from build123d import *

# Parameters (mm, degrees)
SKETCH_1_R          = 1.5
EXTRUDE_1_DEPTH     = 2
EXTRUDE_2_DEPTH     = 17.8
EXTRUDE_3_DEPTH     = 1
CUT_EXTRUDE_START   = 1
CUT_EXTRUDE_1_DEPTH = 13
SKETCH_5_W          = 0.8
SKETCH_5_H          = 3.8
EXTRUDE_4_DEPTH     = 13
SKETCH_6_W          = 4
SKETCH_6_H          = 1
EXTRUDE_5_DEPTH     = 18


with BuildPart() as part:
    # 草图1 → 凸台-拉伸1 (new body)
    with BuildSketch(Plane(origin=(0, 0, 0), x_dir=(1, 0, 0), z_dir=(0, 1, 0))):
        with BuildLine():
            Line((-24.216959088, 1.570750156), (-14.242466434, 28.34905559))
            ThreePointArc((-14.242466434, 28.34905559), (-13.875866128, 28.821296411), (-13.305364415, 29))
            Line((-13.305364415, 29), (13.305364415, 29))
            ThreePointArc((13.305364415, 29), (13.875866128, 28.821296411), (14.242466434, 28.34905559))
            Line((14.242466434, 28.34905559), (24.216959088, 1.570750156))
            ThreePointArc((24.216959088, 1.570750156), (24.5, 0), (24.216959088, -1.570750156))
            Line((24.216959088, -1.570750156), (14.242466434, -28.34905559))
            ThreePointArc((14.242466434, -28.34905559), (13.875866128, -28.821296411), (13.305364415, -29))
            Line((13.305364415, -29), (-13.305364415, -29))
            ThreePointArc((-13.305364415, -29), (-13.875866128, -28.821296411), (-14.242466434, -28.34905559))
            Line((-14.242466434, -28.34905559), (-24.216959088, -1.570750156))
            ThreePointArc((-24.216959088, -1.570750156), (-24.5, 0), (-24.216959088, 1.570750156))
        make_face()
        with Locations((-20, 0)):
            Circle(SKETCH_1_R, mode=Mode.SUBTRACT)
        with Locations((20, 0)):
            Circle(SKETCH_1_R, mode=Mode.SUBTRACT)
    extrude(amount=EXTRUDE_1_DEPTH)

    # 草图2 → 凸台-拉伸2 (add)
    with BuildSketch(Plane.XZ):
        with BuildLine():
            Line((-13.3, -19.3), (-9.3, -23.3))
            Line((-9.3, -23.3), (9.3, -23.3))
            Line((9.3, -23.3), (13.3, -19.3))
            Line((13.3, -19.3), (13.3, 21.3))
            ThreePointArc((13.3, 21.3), (12.714213562, 22.714213562), (11.3, 23.3))
            Line((11.3, 23.3), (-11.3, 23.3))
            ThreePointArc((-11.3, 23.3), (-12.714213562, 22.714213562), (-13.3, 21.3))
            Line((-13.3, 21.3), (-13.3, -19.3))
        make_face()
    extrude(amount=EXTRUDE_2_DEPTH)

    # 草图4 → 凸台-拉伸3 (add)
    with BuildSketch(Plane(origin=(0, 2, 0), x_dir=(1, 0, 0), z_dir=(0, 1, 0))):
        with BuildLine():
            Line((-10.25, 27.15), (10.25, 27.15))
            ThreePointArc((10.25, 27.15), (13.078427125, 25.978427125), (14.25, 23.15))
            Line((14.25, 23.15), (14.25, -23.15))
            ThreePointArc((14.25, -23.15), (13.078427125, -25.978427125), (10.25, -27.15))
            Line((10.25, -27.15), (-10.25, -27.15))
            ThreePointArc((-10.25, -27.15), (-13.078427125, -25.978427125), (-14.25, -23.15))
            Line((-14.25, -23.15), (-14.25, 23.15))
            ThreePointArc((-14.25, 23.15), (-13.078427125, 25.978427125), (-10.25, 27.15))
        make_face()
    extrude(amount=EXTRUDE_3_DEPTH)

    # 草图3 → 切除-拉伸1 (cut)
    with BuildSketch(Plane(origin=(0, 2, 0), x_dir=(1, 0, 0), z_dir=(0, 1, 0)).offset(CUT_EXTRUDE_START)):
        with BuildLine():
            Line((-9, 20.034278181), (9, 20.034278181))
            Line((9, 20.034278181), (12, 17.034278181))
            Line((12, 17.034278181), (12, 4.034278181))
            ThreePointArc((12, 4.034278181), (11.707106781, 3.327171399), (11, 3.034278181))
            Line((11, 3.034278181), (-11, 3.034278181))
            ThreePointArc((-11, 3.034278181), (-11.707106781, 3.327171399), (-12, 4.034278181))
            Line((-12, 4.034278181), (-12, 17.034278181))
            Line((-12, 17.034278181), (-9, 20.034278181))
        make_face()
    extrude(amount=-CUT_EXTRUDE_1_DEPTH, mode=Mode.SUBTRACT)

    # 草图5 → 凸台-拉伸4 (add)
    with BuildSketch(Plane(origin=(0, -10, 0), x_dir=(1, 0, 0), z_dir=(0, 1, 0))):
        with Locations((-7, 9.698034266)):
            Rectangle(SKETCH_5_W, SKETCH_5_H)
        with Locations((0, 13.698034266)):
            Rectangle(SKETCH_5_W, SKETCH_5_H)
        with Locations((7, 9.698034266)):
            Rectangle(SKETCH_5_W, SKETCH_5_H)
    extrude(amount=EXTRUDE_4_DEPTH)

    # 草图6 → 凸台-拉伸5 (add)
    with BuildSketch(Plane.XZ.offset(17.8)):
        with Locations((7.3, 20.63986364)):
            Rectangle(SKETCH_6_W, SKETCH_6_H)
        with Locations((-6.7, 20.63986364)):
            Rectangle(SKETCH_6_W, SKETCH_6_H)
        with Locations((7.3, 15.63986364)):
            Rectangle(SKETCH_6_W, SKETCH_6_H)
        with Locations((-6.7, 15.63986364)):
            Rectangle(SKETCH_6_W, SKETCH_6_H)
        with Locations((7.3, -2.659527469)):
            Rectangle(SKETCH_6_W, SKETCH_6_H)
        with Locations((7.3, -14.202737865)):
            Rectangle(SKETCH_6_W, SKETCH_6_H)
        with Locations((0.634367625, -18.047402207)):
            Rectangle(SKETCH_6_W, SKETCH_6_H)
    extrude(amount=EXTRUDE_5_DEPTH)


solid = part.part
Verification items for the finished model (mm, model axes). A direction names the side the tool comes from. Give positions to 0.01 mm unless a question says otherwise; leave off trailing zeros. Order: outer loops, then holes, each group sorted by start corner. A loop starts at its lowest first (then second) coordinate and runs counter-clockwise, first axis right, second up. Notation, with made-up numbers: M 71,-4 L 86,-4 A15 ccw 86,9 Z; hole C 4,26.25 d4. An arc over 180 degrees is marked long. Use one line per item in the form item = value. Start each with the question number.
Q1. Access from +Z, -Z, +X, -X, +Y, -Y to the whole of each face (thin tool, end or side, straight path). Record for faces 4 (the flat face through (-7, -27, 21.14)), 5 (the flat face through (-7, -27, 20.14)), 6 (the flat face through (11.3, -8.8, -21.3)), 7 (the cylindrical face through (13.047, 2.493, -26.009)), 8 (the flat face through (0, -3, -3.034)).
Q2. Go/stop test with flat-tipped pins: pin 1 Ø0.5 at (y, z) = (-22.5, 20.5) entering from +X; pin 2 Ø1.9 at (y, z) = (-3, -10) entering from +X; pin 3 Ø5 at (x, z) = (-17, 11) entering from -Y; pin 4 Ø8 at (y, z) = (-26, -9) entering from +X. Record where each tip stops, or that it passes through.
Q3. Section check A-A (y = -22). Enter the section's corners in (x, z), then the cut area to 3 significant figures.
Q4. Section check D-D (x = 20). Enter the section's corners in (y, z).
Q5. Scan lines: line 1 along Z through (x, y) = (-6, -19); line 2 along X through (y, z) = (1.5, 1); line 3 along Y through (x, z) = (11, 2.5). Record each from-to range of solid material in increasing order. Write a range as [from, to].
Q6. Section check B-B (z = 0). Enter the section's corners in (x, y), then the cut area to 3 significant figures.
Q7. Mould release check, pull along X, two halves, no side actions. Record for faces 1 (the cylindrical face through (-13.047, 2.493, 26.009)), 2 (the flat face through (-7, -27, 15.14)), 3 (the flat face through (-12, -3, -10)): +X half, -X half, draft (parallel to the pull), parting line (faces both ways), or undercut.
Q8. Section check C-C (y = -8). Enter the section's corners in (x, z), then the cut area to 3 significant figures.
Evaluation:
q1.face_4 = +Z, +X, -X, -Y
q1.face_5 = +X, -X, -Y
q1.face_6 = -Z, +X, -Y
q1.face_7 = -Z, +X, +Y
q1.face_8 = +Y
q2.pin_1 = 9.3
q2.pin_2 = 13.3
q2.pin_3 = 0
q2.pin_4 = through
q3.outline = M -8.7,15.14 L -4.7,15.14 L -4.7,16.14 L -8.7,16.14 Z; M -8.7,20.14 L -4.7,20.14 L -4.7,21.14 L -8.7,21.14 Z; M -1.37,-18.55 L 2.63,-18.55 L 2.63,-17.55 L -1.37,-17.55 Z; M 5.3,-14.7 L 9.3,-14.7 L 9.3,-13.7 L 5.3,-13.7 Z; M 5.3,-3.16 L 9.3,-3.16 L 9.3,-2.16 L 5.3,-2.16 Z; M 5.3,15.14 L 9.3,15.14 L 9.3,16.14 L 5.3,16.14 Z; M 5.3,20.14 L 9.3,20.14 L 9.3,21.14 L 5.3,21.14 Z
q3.area = 28.0 mm2
q4.outline = M 0,-12.89 L 2,-12.89 L 2,-1.5 L 0,-1.5 Z; M 0,1.5 L 2,1.5 L 2,12.89 L 0,12.89 Z
q5.line_1 = [15.14, 16.14], [20.14, 21.14]
q5.line_2 = [-24.39, -21.12], [-18.88, 18.88], [21.12, 24.39]
q5.line_3 = [-17.8, 3]
q6.outline = M -24.5,0 L -21.5,0 L -21.5,2 L -24.5,2 Z; M -18.5,0 L -13.3,0 L -13.3,-17.8 L 13.3,-17.8 L 13.3,0 L 18.5,0 L 18.5,2 L 14.25,2 L 14.25,3 L -14.25,3 L -14.25,2 L -18.5,2 Z; M 21.5,0 L 24.5,0 L 24.5,2 L 21.5,2 Z
q6.area = 588 mm2
q7.face_1 = -X half
q7.face_2 = draft
q7.face_3 = undercut
q8.outline = M -13.3,-19.3 L -9.3,-23.3 L 9.3,-23.3 L 13.3,-19.3 L 13.3,21.3 A2 ccw 11.3,23.3 L -11.3,23.3 A2 ccw -13.3,21.3 Z; M -7.4,-11.6 L -6.6,-11.6 L -6.6,-7.8 L -7.4,-7.8 Z; M -0.4,-15.6 L 0.4,-15.6 L 0.4,-11.8 L -0.4,-11.8 Z; M 6.6,-11.6 L 7.4,-11.6 L 7.4,-7.8 L 6.6,-7.8 Z; hole M -12,-17.03 L -9,-20.03 L 9,-20.03 L 12,-17.03 L 12,-4.03 A1 ccw 11,-3.03 L -11,-3.03 A1 ccw -12,-4.03 Z
q8.area = 832 mm2
